Job drawing, mm, ordinate dimensions from the low corner. One solid piece. Give positions to 0.01 mm unless a question says otherwise; leave off trailing zeros. Loops run counter-clockwise (first coordinate to the right, second up) from the corner with the lowest first, then second, coordinate; pieces in that order, holes last. Notation, with made-up numbers: (48, 0) -> (97, 0) arc R33 ccw to (97, 34) -> close; hole circle Ø4 at (32, 64.5). An arc over 180 degrees is marked (long way). Use one line per item in the form item = value.
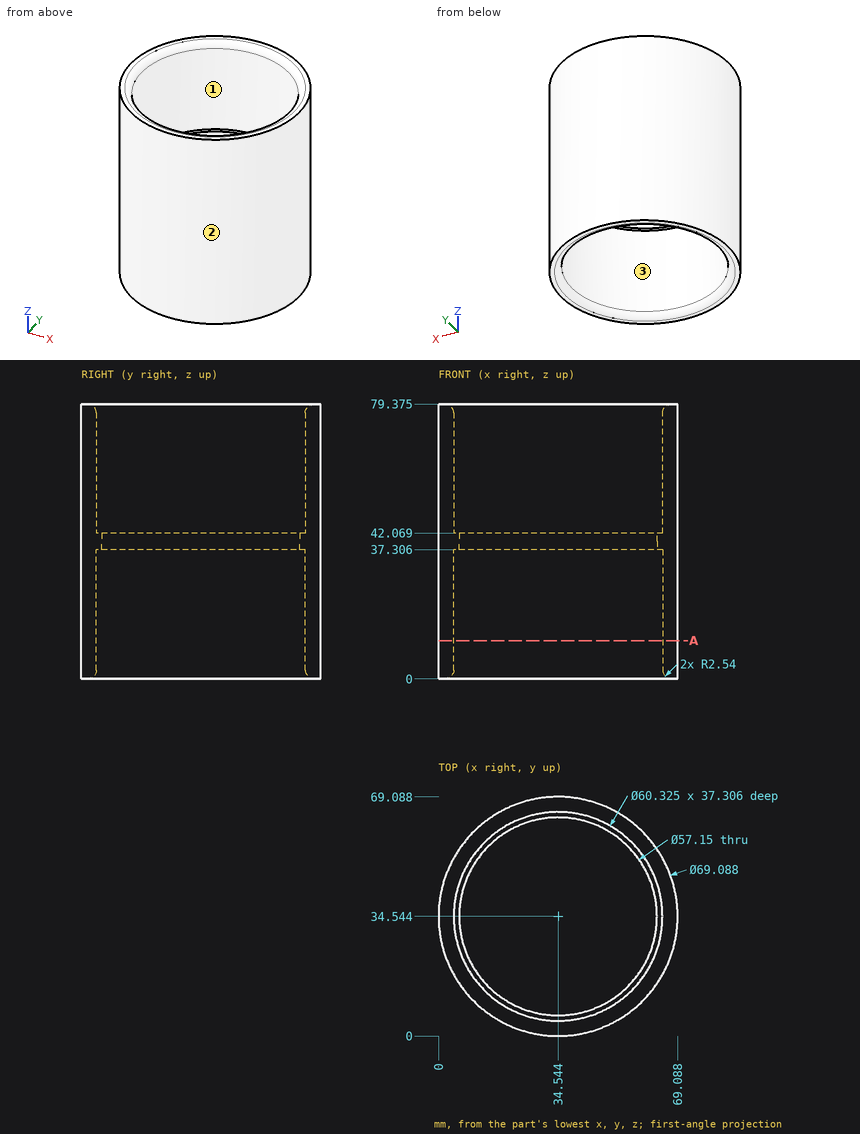
1. Drill centre lines: line 1 (Y direction, x = 58, z = 67) (1 decimal); line 2 (Z direction, x = 39.5, y = 63); line 3 (Y direction, x = 32, z = 49). Where is each one in solid material? Low to high.
Result sheet:
line_1 = 9.2 to 15.6, 53.5 to 59.9
line_2 = 37.31 to 42.07
line_3 = 0.09 to 4.49, 64.6 to 68.99
2. Drop flat-ended pins along their axis: P1, Ø10, axis at x = 29.5, z = 43.5, coming from the -Y side; P2, Ø3, axis at y = 22.5, z = 49, coming from the -X side; P3, Ø1.5, axis at x = 27.5, z = 27, coming from the +Y side. Give the stop position or say it passes through.
Result sheet:
P1 = 0
P2 = 1.65
P3 = 68.51
3. Cut at A-A, the plane z = 11. Write the cut outline in (x, y) (1 decimal).
Result sheet:
outline = circle Ø69.1 at (34.5, 34.5); hole circle Ø60.3 at (34.5, 34.5)
4. Mould opens along Y. For the marked faces 1, 2 and 3 say: pulls with the +Y half, pulls with the -Y half, needs draft (parallel to the pull), parting line crosses it, or undercut.
Result sheet:
face_1 = undercut
face_2 = parting line crosses it
face_3 = undercut
